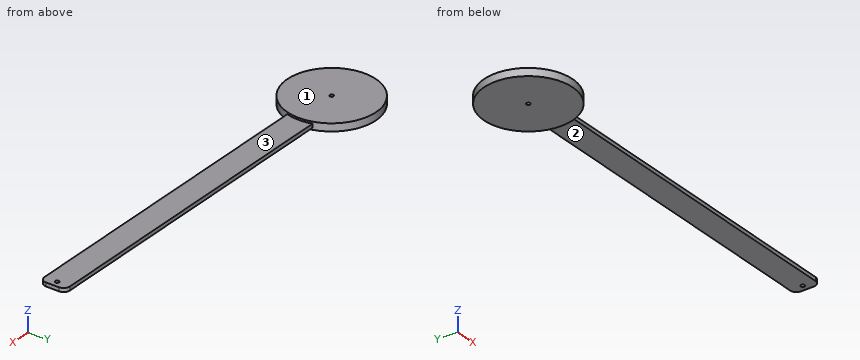
from build123d import *

# Parameters (mm, degrees)
SKETCH1_R                = 1.5
BOSS_EXTRUDE1_DEPTH      = 3
BOSS_EXTRUDE2_DEPTH      = 3
BOSS_EXTRUDE2_DEPTH_BACK = 3
BOSS_EXTRUDE2_START      = 1.5
SKETCH4_R                = 35
SKETCH9_R                = 1.5
CUT_EXTRUDE1_DEPTH       = 184.469343488


with BuildPart() as part:
    # Sketch1 → Boss-Extrude1 (new body)
    with BuildSketch(Plane.XY):
        with BuildLine():
            Line((-145, 10), (145, 10))
            ThreePointArc((145, 10), (148.535533906, 8.535533906), (150, 5))
            Line((150, 5), (150, -5))
            ThreePointArc((150, -5), (148.535533906, -8.535533906), (145, -10))
            Line((145, -10), (-145, -10))
            ThreePointArc((-145, -10), (-148.535533906, -8.535533906), (-150, -5))
            Line((-150, -5), (-150, 5))
            ThreePointArc((-150, 5), (-148.535533906, 8.535533906), (-145, 10))
        make_face()
        with Locations((145, 0)):
            Circle(SKETCH1_R, mode=Mode.SUBTRACT)
    extrude(amount=BOSS_EXTRUDE1_DEPTH)

    # Sketch4 → Boss-Extrude2 (add, two sides: drawn at the far end of the back side and taken through both)
    with BuildSketch(Plane.XY.offset(BOSS_EXTRUDE2_START - BOSS_EXTRUDE2_DEPTH_BACK)):
        with Locations((-145, 0)):
            Circle(SKETCH4_R)
    extrude(amount=BOSS_EXTRUDE2_DEPTH + BOSS_EXTRUDE2_DEPTH_BACK)

    # Sketch9 → Cut-Extrude1 (cut, through all)
    with BuildSketch(Plane.XY.offset(4.5)):
        with Locations((-145, 0)):
            Circle(SKETCH9_R)
    extrude(amount=-CUT_EXTRUDE1_DEPTH, mode=Mode.SUBTRACT)


solid = part.part
Here's how the part is built. I have some questions about the finished solid (model axes, mm). Face numbers are marked on the shaded views. A direction names the side the tool comes from. Round coordinates to 2 decimals unless told otherwise and drop trailing zeros. Write each loop counter-clockwise with the first axis right and the second up, starting at its lowest first coordinate (ties: lowest second). Pieces come first, ordered by that corner, then holes. Notation, with made-up numbers: (-37, -3) -> (-24, -3) arc R15 ccw to (-24, 20) -> close; hole circle Ø3 at (21, 45). An arc over 180 degrees is marked (long way). One line per item, written item: value.
1) Suppose I cut it at A-A on x = 125. List the corners of the cut face in (y, z) for me.
Filled sheet:
outline: (-10, 0) -> (10, 0) -> (10, 3) -> (-10, 3) -> close
2) I'm going to push flat-ended pins straight in: pin 1 Ø4 at (x, y) = (145, 0) entering from -Z; pin 2 Ø1 at (x, z) = (-125.5, 1) entering from +Y; pin 3 Ø2 at (y, z) = (17, -0.5) entering from +X; pin 4 Ø2.5 at (x, y) = (-145, 0) entering from +Z (1 decimal). Where does each tip first touch, or does it pass through?
Filled sheet:
pin 1: stops at z = 0
pin 2: stops at y = 29.39
pin 3: stops at x = -113.87
pin 4: passes through
3) If I drill on line 1 (Y direction, x = -145, z = -0.25); line 2 (Z direction, x = -103.5, y = 8); line 3 (Y direction, x = 13, z = 1.3), over which ranges is the centre line in solid material (lowest first)? Write a range as [from, to].
Filled sheet:
line 1: y = [-35, -1.5], [1.5, 35]
line 2: z = [0, 3]
line 3: y = [-10, 10]
4) For the marked faces 1, 2 and 3, which set-ups out of +Z, -Z, +X, -X, +Y, -Y let a thin tool reach every point of the face, with its end or its side?
Filled sheet:
face 1: +Z, +X, -X, +Y, -Y
face 2: -Z, +X, +Y, -Y
face 3: +Z, +X, +Y, -Y
5) Suppose I cut it at B-B on y = 28.5. List the corners of the cut face in (x, z) for me, plus the area to 3 significant figures.
Filled sheet:
outline: (-165.32, -1.5) -> (-124.68, -1.5) -> (-124.68, 4.5) -> (-165.32, 4.5) -> close
area: 244 mm2
